```python
from build123d import *

# Parameters (mm, degrees)
ESTRUSIONE_ESTRUSIONE1_DEPTH = 6
SCHIZZO2_R                   = 12.5
ESTRUSIONE_ESTRUSIONE2_DEPTH = 16
FORO1_D                      = 1.75
FORO1_CSINK_D                = 6
FORO1_CSINK_ANGLE            = 82


with BuildPart() as part:
    # Schizzo1 → Estrusione-Estrusione1 (new body)
    with BuildSketch(Plane.XY):
        Polygon((0, 17.320508076), (-15, 8.660254038), (-15, -8.660254038), (0, -17.320508076), (15, -8.660254038), (15, 8.660254038), align=None)
    extrude(amount=ESTRUSIONE_ESTRUSIONE1_DEPTH)

    # Schizzo2 → Estrusione-Estrusione2 (add)
    with BuildSketch(Plane.XY.offset(6)):
        Circle(SCHIZZO2_R)
    extrude(amount=ESTRUSIONE_ESTRUSIONE2_DEPTH)

    # Foro1 (through all)
    with Locations(Plane.XY.offset(22)):
        with Locations((0, 0)):
            CounterSinkHole(FORO1_D / 2, FORO1_CSINK_D / 2, counter_sink_angle=FORO1_CSINK_ANGLE)

    # Schizzo7 → Taglia-Rivoluzione1 (revolve, cut)
    with BuildSketch(Plane(origin=(0, 0, 0), x_dir=(1, 0, 0), z_dir=(0, 1, 0))):
        Polygon((-1.5, 0), (0, -1.5), (0, 0), align=None)
    revolve(axis=Axis((0, 0, 1.5), (0, 0, -1)), mode=Mode.SUBTRACT)


solid = part.part
```
Can you work these out from the model? Positions are in its coordinate system, mm. A direction names the side the tool comes from. Coordinates: 2 decimals unless noted, no trailing zeros. Loops run counter-clockwise (first coordinate to the right, second up) from the corner with the lowest first, then second, coordinate; pieces in that order, holes last. Notation, with made-up numbers: M 17,-2 L 55,-2 A27 cw 55,24 Z; hole C 68.5,-40 d10. An arc over 180 degrees is marked long. Put each result on its own line as item: value. Start each with the question number.
(1) We'd pull the mould along X, two halves only. Please class faces 3 (the face through (-15, 0, 3)), 4 (the face through (-0.93, 0.29, 19.67)), 5 (the face through (7.4, -13.05, 2.96)): +X half, -X half, draft (parallel to the pull), parting line (faces both ways), or undercut.
(2) Imagine slicing it at B-B on y = 0. List the corners of the cut face in (x, z) for me (3 decimals).
(3) Will these pins go through, and if not, where does the flat tip stop? pin 1 Ø5 at (x, z) = (-10, 4) entering from +Y; pin 2 Ø3 at (x, y) = (-8.5, -12) entering from +Z; pin 3 Ø3 at (y, z) = (11.5, 13) entering from +X; pin 4 Ø1.6 at (x, y) = (0, 0) entering from +Z.
(4) Imagine slicing it at D-D on x = 6. List the corners of the cut face in (y, z) for me, and give its area (3 significant figures).
(5) Which directions (+Z, -Z, +X, -X, +Y, -Y) give clear straight access to the entire face, cutting with the end or side of a thin tool? Please do faces 1 (the face through (0, -4, 0)), 2 (the face through (0, -13, 6)).
(6) Imagine slicing it at C-C on y = 6. List the corners of the cut face in (x, z) for me.
(7) I need wall thicknesses on probe 1 along Y at (x, z) = (0, 13) (3 decimals); probe 2 along Y at (x, z) = (0, 4.5) (1 decimal); probe 3 along Z at (x, y) = (0.25, -14.5). Which ranges of each line are inside material? Lowest first, please.
Worked answers:
1. face 3: -X half
1. face 4: undercut
1. face 5: +X half
2. outline: M -15,0 L -1.5,0 L -0.875,0.625 L -0.875,19.555 L -3,22 L -12.5,22 L -12.5,6 L -15,6 Z; M 0.875,0.625 L 1.5,0 L 15,0 L 15,6 L 12.5,6 L 12.5,22 L 3,22 L 0.875,19.555 Z
3. pin 1: stops at y = 12.99
3. pin 2: stops at z = 6
3. pin 3: stops at x = 7.5
3. pin 4: passes through
4. outline: M -13.86,0 L 13.86,0 L 13.86,6 L 10.97,6 L 10.97,22 L -10.97,22 L -10.97,6 L -13.86,6 Z
4. area: 517 mm2
5. face 1: -Z, +X, -X, +Y, -Y
5. face 2: +Z
6. outline: M -15,0 L 15,0 L 15,6 L 10.97,6 L 10.97,22 L -10.97,22 L -10.97,6 L -15,6 Z
7. probe 1: y = -12.5 to -0.875, 0.875 to 12.5
7. probe 2: y = -17.3 to -0.9, 0.9 to 17.3
7. probe 3: z = 0 to 6
